Input: part model. Units: mm. Frame: model coordinates. Face numbers are marked on the shaded views. A direction names the side the tool comes from. Give positions to 0.01 mm unless a question says otherwise; leave off trailing zeros. Loops run counter-clockwise (first coordinate to the right, second up) from the corner with the lowest first, then second, coordinate; pieces in that order, holes last. Notation, with made-up numbers: M -34,61.25 L 20,61.25 A23 cw 20,76.25 Z; hole C 51,22.25 d8. An arc over 180 degrees is marked long. One line per item, written item: value. Start each with the question number.
(1) Section B-B on y = -75. Output: boundary loops of the cut face in (x, z).
(2) Pin query (flat end, axial travel): P1, Ø8, axis at x = -12, y = -102, coming from the +Z side; P2, Ø4, axis at x = -30, y = -76, coming from the -Z side; P3, Ø5.5, axis at x = -39.5, y = -75, coming from the +Z side. Return the tip coordinate at first contact, or that it passes through.
(3) Access query for the marked faces 1, 2 and 3. Directions: +Z, -Z, +X, -X, +Y, -Y. A direction counts if a zero-diameter tool reaches every point of the face in a straight line with its end or side. Return the directions, or none.
(4) Section A-A on x = 0. Output: boundary loops of the cut face in (y, z).
(5) Section D-D on x = -37.3. Output: boundary loops of the cut face in (y, z).
(6) Section C-C on z = 0. Output: boundary loops of the cut face in (x, y), plus the area to 3 significant figures.
(7) Ray query, line 1 along X through (y, z) = (-27, -0.25); line 2 along Z through (x, y) = (-37.3, -61.5); line 3 along Z through (x, y) = (0, -97). Return the intervals inside material, ascending. Write a range as from..to.
```python
from build123d import *

# Parameters (mm, degrees)
F0_R     = 5.1
F0_R_2   = 4.1
F1_DEPTH = 160


with BuildPart() as f1:
    # F0 (on Front) → F1 (new body)
    with BuildSketch(Plane.XZ):
        with BuildLine():
            ThreePointArc((-9.219544, -4), (-8.266082, -4.241902), (-7.543264, -4.909091))
            ThreePointArc((-7.543264, -4.909091), (9, 0), (-7.543264, 4.909091))
            ThreePointArc((-7.543264, 4.909091), (-8.266082, 4.241902), (-9.219544, 4))
            Line((-9.219544, 4), (-19.475736, 4))
            ThreePointArc((-19.475736, 4), (-19.590541, 3.977164), (-19.687868, 3.912132))
            Line((-19.687868, 3.912132), (-20.1, 3.5))
            Line((-20.1, 3.5), (-20.512132, 3.912132))
            ThreePointArc((-20.512132, 3.912132), (-20.609459, 3.977164), (-20.724264, 4))
            Line((-20.724264, 4), (-28.821652, 4))
            ThreePointArc((-28.821652, 4), (-30.522492, 4.528737), (-31.623801, 5.928571))
            ThreePointArc((-31.623801, 5.928571), (-33.092213, 7.795018), (-35.36, 8.5))
            Line((-35.36, 8.5), (-42.3, 8.5))
            ThreePointArc((-42.3, 8.5), (-44.42132, 7.62132), (-45.3, 5.5))
            Line((-45.3, 5.5), (-45.3, -5.5))
            ThreePointArc((-45.3, -5.5), (-44.42132, -7.62132), (-42.3, -8.5))
            Line((-42.3, -8.5), (-35.36, -8.5))
            ThreePointArc((-35.36, -8.5), (-33.092213, -7.795018), (-31.623801, -5.928571))
            ThreePointArc((-31.623801, -5.928571), (-30.522492, -4.528737), (-28.821652, -4))
            Line((-28.821652, -4), (-20.724264, -4))
            ThreePointArc((-20.724264, -4), (-20.609459, -3.977164), (-20.512132, -3.912132))
            Line((-20.512132, -3.912132), (-20.1, -3.5))
            Line((-20.1, -3.5), (-19.687868, -3.912132))
            ThreePointArc((-19.687868, -3.912132), (-19.590541, -3.977164), (-19.475736, -4))
            Line((-19.475736, -4), (-9.219544, -4))
        make_face()
        with Locations((-37.3, 0)):
            Circle(F0_R, mode=Mode.SUBTRACT)
        Circle(F0_R_2, mode=Mode.SUBTRACT)
    extrude(amount=F1_DEPTH)


solid = f1.part
```
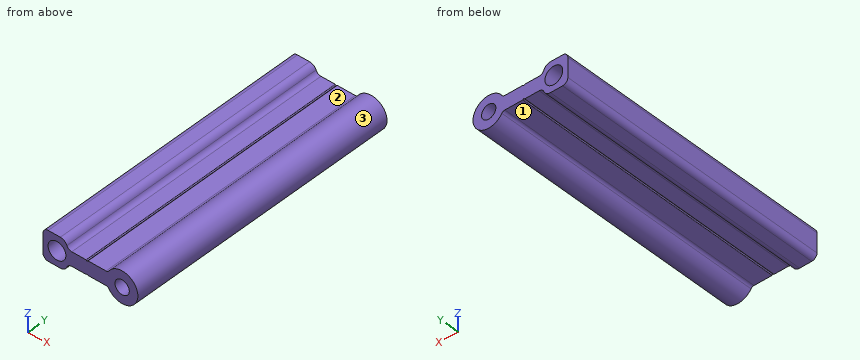
Output values:
1. outline: M -45.3,-5.5 A3 ccw -42.3,-8.5 L -35.36,-8.5 A4 ccw -31.62,-5.93 A3 cw -28.82,-4 L -20.72,-4 A0.3 ccw -20.51,-3.91 L -20.1,-3.5 L -19.69,-3.91 A0.3 ccw -19.48,-4 L -9.22,-4 A2 cw -7.54,-4.91 A9 ccw long -7.54,4.91 A2 cw -9.22,4 L -19.48,4 A0.3 ccw -19.69,3.91 L -20.1,3.5 L -20.51,3.91 A0.3 ccw -20.72,4 L -28.82,4 A3 cw -31.62,5.93 A4 ccw -35.36,8.5 L -42.3,8.5 A3 ccw -45.3,5.5 Z; hole C -37.3,0 d10.2; hole C 0,0 d8.2
2. P1: stops at z = 4.41
2. P2: stops at z = -6.67
2. P3: stops at z = 8.5
3. face 1: -Z, +Y, -Y
3. face 2: +Z, +Y, -Y
3. face 3: +Y, -Y
4. outline: M -160,-9 L 0,-9 L 0,-4.1 L -160,-4.1 Z; M -160,4.1 L 0,4.1 L 0,9 L -160,9 Z
5. outline: M -160,-8.5 L 0,-8.5 L 0,-5.1 L -160,-5.1 Z; M -160,5.1 L 0,5.1 L 0,8.5 L -160,8.5 Z
6. outline: M -45.3,-160 L -42.4,-160 L -42.4,0 L -45.3,0 Z; M -32.2,-160 L -4.1,-160 L -4.1,0 L -32.2,0 Z; M 4.1,-160 L 9,-160 L 9,0 L 4.1,0 Z
6. area: 5,740 mm²
7. line 1: x = -45.3..-42.39, -32.21..-4.09, 4.09..9
7. line 2: z = -8.5..-5.1, 5.1..8.5
7. line 3: z = -9..-4.1, 4.1..9
